Autodesk Inventor part; units mm, degrees
ref_plane "YZ Plane" through (0, 0, 0) normal (1, 0, 0) x (0, 1, 0)
ref_plane "XZ Plane" through (0, 0, 0) normal (0, 1, 0) x (-1, 0, 0)
ref_plane "XY Plane" through (0, 0, 0) normal (0, 0, 1) x (1, 0, 0)
sketch "Szkic1" plane through (0, 0, 0) normal (0, 1, 0) x (-1, 0, 0)
  line L0 (40, -30) -> (25, -30)
  line L1 (-45, -25) -> (-45, 25)
  line L2 (-40, 30) -> (-25, 30)
  line L3 (45, 25) -> (45, -25)
  arc A0 (45, 25) -> (40, 30) centre (40, 25) ccw
  arc A1 (40, -30) -> (45, -25) centre (40, -25) ccw
  arc A2 (-45, -25) -> (-40, -30) centre (-40, -25) ccw
  arc A3 (-40, 30) -> (-45, 25) centre (-40, 25) ccw
  line L4 (40, 30) -> (35, 30)
  line L5 (20, 30) -> (20, 25)
  line L6 (20, 25) -> (25, 25)
  line L7 (25, 25) -> (25, 30)
  line L8 (2.5, 30) -> (-2.5, 30)
  line L9 (-25, 30) -> (-25, 25)
  line L10 (-25, 25) -> (-20, 25)
  line L11 (-20, 25) -> (-20, 30)
  line L12 (-35, 30) -> (-40, 30)
  line L13 (35, -30) -> (40, -30)
  line L14 (25, -25) -> (20, -25)
  line L15 (20, -25) -> (20, -30)
  line L16 (25, -30) -> (25, -25)
  line L17 (-2.5, -30) -> (2.5, -30)
  line L18 (-20, -25) -> (-25, -25)
  line L19 (-25, -25) -> (-25, -30)
  line L20 (-20, -30) -> (-20, -25)
  line L21 (-40, -30) -> (-35, -30)
  line L22 (20, -30) -> (-20, -30)
  line L23 (-25, -30) -> (-40, -30)
  line L24 (-20, 30) -> (20, 30)
  line L25 (25, 30) -> (40, 30)
  point P0 (0, 0)
  point P1 (40, -30)
  dimension "d2" = 5
  dimension "d5" = 5
  dimension "d6" = 5
  dimension "d9" = 5
  dimension "d12" = 5
  dimension "d13" = 5
  dimension "d15" = 5
  dimension "d17" = 5
  dimension "d19" = 5
  dimension "d21" = 5
ref_plane "Płaszczyzna konstrukcyjna2" through (0, 0, 0) normal (0, -1, 0) x (1, 0, 0)
sketch "Szkic5" plane through (0, 0, 0) normal (0, -1, 0) x (1, 0, 0)
  line L0 (25, 25) -> (20, 25)
  line L1 (20, 25) -> (20, 40)
  line L2 (20, 40) -> (25, 40)
  line L3 (25, 40) -> (25, 25)
  line L4 (-20, 25) -> (-25, 25)
  line L5 (-25, 25) -> (-25, 40)
  line L6 (-25, 40) -> (-20, 40)
  line L7 (-20, 40) -> (-20, 25)
  line L8 (25, -25) -> (20, -25)
  line L9 (20, -25) -> (20, -40)
  line L10 (20, -40) -> (25, -40)
  line L11 (25, -40) -> (25, -25)
  line L12 (-20, -25) -> (-25, -25)
  line L13 (-25, -25) -> (-25, -40)
  line L14 (-25, -40) -> (-20, -40)
  line L15 (-20, -40) -> (-20, -25)
  point P0 (0, 0)
  dimension "d56" = 5
  dimension "d57" = 15
  dimension "d58" = 5
  dimension "d59" = 15
  dimension "d60" = 5
  dimension "d61" = 15
  dimension "d62" = 5
  dimension "d63" = 15
extrude "Wyciągnięcie proste5" add sketch "Szkic5" against normal blind 5
ref_plane "Płaszczyzna konstrukcyjna3" through (0, 5, 0) normal (0, 1, 0) x (1, 0, 0)
sketch "Szkic6" plane through (0, 5, 0) normal (0, 1, 0) x (1, 0, 0)
  line L0 (25, -40) -> (20, -40)
  line L1 (20, -40) -> (20, -35)
  line L2 (20, -35) -> (25, -35)
  line L3 (25, -35) -> (25, -40)
  line L4 (-20, -40) -> (-25, -40)
  line L5 (-25, -40) -> (-25, -35)
  line L6 (-25, -35) -> (-20, -35)
  line L7 (-20, -35) -> (-20, -40)
  line L8 (25, 40) -> (20, 40)
  line L9 (20, 40) -> (20, 35)
  line L10 (20, 35) -> (25, 35)
  line L11 (25, 35) -> (25, 40)
  line L12 (-20, 40) -> (-25, 40)
  line L13 (-25, 40) -> (-25, 35)
  line L14 (-25, 35) -> (-20, 35)
  line L15 (-20, 35) -> (-20, 40)
  point P0 (0, 0)
  dimension "d64" = 5
  dimension "d66" = 5
  dimension "d67" = 5
  dimension "d68" = 5
  dimension "d69" = 5
  dimension "d70" = 5
  dimension "d71" = 5
  dimension "d72" = 5
  dimension "d73" = 5
extrude "Wyciągnięcie proste6" add sketch "Szkic6" along normal blind 20
extrude "Wyciągnięcie proste7" add sketch "Szkic1" along normal blind 5
sketch "Szkic7" plane through (0, 0, 0) normal (0, -1, 0) x (1, 0, 0)
  point P0 (0, 0)
properties part number "Floor"
Build history of the part. All positions in model axes, mm. A direction names the side the tool comes from. Give positions to 0.01 mm unless a question says otherwise; leave off trailing zeros. Loops run counter-clockwise (first coordinate to the right, second up) from the corner with the lowest first, then second, coordinate; pieces in that order, holes last.
Item 1: Pull direction Z, two halves, no side cores. Call faces 5 (the face through (22, 12, 40)), 6 (the face through (-20, 10, 36)), 7 (the face through (-23, 15, 35)): released by +Z, released by -Z, zero draft, split by the parting line, or undercut.
Answers follow:
face 5: released by +Z
face 6: zero draft
face 7: undercut
Item 2: Drill centre line: line 1 (Y direction, x = 30.5, z = -27). Where is it in solid material? Low to high.
Answers follow:
line 1: y = 0 to 5
Item 3: Slice it at B-B, the plane z = 31. List the corners of the cut face in (x, y).
Answers follow:
outline: (-25, 0) - (-20, 0) - (-20, 5) - (-25, 5) - close; (20, 0) - (25, 0) - (25, 5) - (20, 5) - close
Item 4: Slice it at A-A, the plane y = 12. List the corners of the cut face in (x, z).
Answers follow:
outline: (-25, -40) - (-20, -40) - (-20, -35) - (-25, -35) - close; (-25, 35) - (-20, 35) - (-20, 40) - (-25, 40) - close; (20, -40) - (25, -40) - (25, -35) - (20, -35) - close; (20, 35) - (25, 35) - (25, 40) - (20, 40) - close
Item 5: Slice it at D-D, the plane x = 30.5. List the corners of the cut face in (y, z).
Answers follow:
outline: (0, -30) - (5, -30) - (5, 30) - (0, 30) - close
Item 6: Slice it at C-C, the plane y = 2.5. List the corners of the cut face in (x, z).
Answers follow:
outline: (-45, -25) arc R5 ccw to (-40, -30) - (-25, -30) - (-25, -40) - (-20, -40) - (-20, -30) - (20, -30) - (20, -40) - (25, -40) - (25, -30) - (40, -30) arc R5 ccw to (45, -25) - (45, 25) arc R5 ccw to (40, 30) - (25, 30) - (25, 40) - (20, 40) - (20, 30) - (-20, 30) - (-20, 40) - (-25, 40) - (-25, 30) - (-40, 30) arc R5 ccw to (-45, 25) - close
Item 7: Flat gauge pins, fed straight in: pin 1 (5 mm diameter, centred on y = 8, z = 33.5, fed in from -X); pin 2 (3 mm diameter, centred on y = 16, z = -36, fed in from +X); pin 3 (2.5 mm diameter, centred on x = 31.5, y = 2.5, fed in from -Z). Where does each tip first touch, or does it go through?
Answers follow:
pin 1: stops at x = -25
pin 2: stops at x = 25
pin 3: stops at z = -30
Item 8: Which spindle directions (+Z, -Z, +X, -X, +Y, -Y) get a long thin tool onto all of the face, cutting with end or side? Do faces 1 (the face through (20, 10, 37)), 2 (the face through (-20, 10, -36)), 3 (the face through (25, 10, 36)), 4 (the face through (25, 10, -36)). Say none if no direction does.
Answers follow:
face 1: +Z, +Y, -Y
face 2: -Z, +Y, -Y
face 3: +Z, +X, +Y, -Y
face 4: -Z, +X, +Y, -Y
